The listing builds one solid part. Answer for the finished solid, in the listing's coordinates (mm). A direction names the side the tool comes from. Give positions to 0.01 mm unless a question says otherwise; leave off trailing zeros. Order: outer loops, then holes, each group sorted by start corner. A loop starts at its lowest first (then second) coordinate and runs counter-clockwise, first axis right, second up. Notation, with made-up numbers: (33.5, -37.75) - (44.5, -37.75) arc R30 cw to (44.5, -12.75) - close; hole circle Ø5 at (60, 80). An arc over 180 degrees is marked (long way). Use a Markdown table: item, result. Add a question column.
1) Find section B-B, the plane x = 13.5. Determine the outline of the cut face in (y, z) (3 decimals), plus the area to 3 significant figures.
2) Straight lines are drawn through the part: line 1 (X direction, y = 1.8, z = -4.65) (3 decimals); line 2 (Z direction, x = -4, y = 1.55) (3 decimals); line 3 (Z direction, x = 13.5, y = 1.65) (3 decimals). For each, find the intervals that lie inside material, in ascending order.
3) Find section C-C, the plane z = 30. Determine the outline of the cut face in (x, y).
4) The mould has two halves that part along X. Classify faces 4 (the face through (-2, 2, 31.5)), 5 (the face through (-14.448, 1.726, -22.078)), 6 (the face through (-14.853, 1.726, -3.946)): released by +X, released by -X, zero draft, split by the parting line, or undercut.
5) Find section A-A, the plane x = -13.5. Determine the outline of the cut face in (y, z) (3 decimals).
6) For faces 1 (the face through (-8.409, 1.774, -6.435)), 2 (the face through (-3.6, 2, 17)), 3 (the face through (19, 2, 15.4)), determine the directions among +Z, -Z, +X, -X, +Y, -Y from which every point of the face is accessible in a straight line to the end or side of a thin tool.
7) Find section D-D, the plane y = 0.8. State how many separate pieces and enclosed holes the cut face has, plus the area to 3 significant figures.
8) Flat-ended cylindrical pins translate along their axes: pin 1 (1 mm diameter, centred on y = 1.5, z = 14, fed in from -X); pin 2 (1.5 mm diameter, centred on y = 1.5, z = -16, fed in from +X); pin 3 (1.8 mm diameter, centred on x = 18.5, y = 1, fed in from -Z). Find the tip coordinate at first contact, or state that the pin passes through.
from build123d import *

# Parameters (mm, degrees)
SKETCH2_R           = 1.525
BOSS_EXTRUDE1_DEPTH = 3.5
FILLET1_R           = 5
FILLET2_R           = 2


with BuildPart() as part:
    # Sketch2 → Boss-Extrude1 (new body)
    with BuildSketch(Plane(origin=(0, 0, 0), x_dir=(1, 0, 0), z_dir=(0, 1, 0))):
        Polygon((-8, 29.459088021), (8, 29.459088021), (20.5, 15.15), (20.5, -13.4), (17, -13.4), (17, -15.4), (20.5, -15.4), (20.5, -18.9), (17, -18.9), (17, -31.5), (20.5, -31.5), (20.5, -35), (17, -35), (17, -37), (-0.1, -37), (-0.1, -35), (-3.6, -35), (-3.6, -31.5), (-0.1, -31.5), (-0.1, -18.9), (-3.6, -18.9), (-3.6, -15.4), (-0.1, -15.4), (-0.1, -13.4), (-3.6, -13.4), (-3.6, 0), (-20.5, 0), (-20.5, 15.15), align=None)
        with Locations(Location((-5.25, 25.459088021, 0), (0, 0, 270))):
            Circle(SKETCH2_R, mode=Mode.SUBTRACT)
        with Locations(Location((-13.5, 4.65, 0), (0, 0, 270))):
            Circle(SKETCH2_R, mode=Mode.SUBTRACT)
        with Locations(Location((13.5, 4.65, 0), (0, 0, 90))):
            Circle(SKETCH2_R, mode=Mode.SUBTRACT)
        with Locations(Location((5.25, 25.459088021, 0), (0, 0, 90))):
            Circle(SKETCH2_R, mode=Mode.SUBTRACT)
        with BuildLine():
            Line((8.711994152, 6.175), (-8.711994152, 6.175))
            ThreePointArc((-8.711994152, 6.175), (-10.168396205, 8.411786963), (-12.564791667, 9.587206738))
            ThreePointArc((-12.564791667, 9.587206738), (0, 18.15), (12.564791667, 9.587206738))
            ThreePointArc((12.564791667, 9.587206738), (10.168396205, 8.411786963), (8.711994152, 6.175))
        make_face(mode=Mode.SUBTRACT)
        with BuildLine():
            ThreePointArc((4.678763834, -20.194315192), (8.45, -25.527648525), (12.221236166, -20.194315192))
            ThreePointArc((12.221236166, -20.194315192), (8.45, -9.527648525), (4.678763834, -20.194315192))
        make_face(mode=Mode.SUBTRACT)
    extrude(amount=BOSS_EXTRUDE1_DEPTH)

    # Fillet1
    fillet1_edges = [part.edges().sort_by_distance(p)[0] for p in [
        (20.5, 1.75, -15.15),
        (-3.6, 1.75, 0),
        (-20.5, 1.75, 0),
        (-20.5, 1.75, -15.15),
        (-8, 1.75, -29.459088021),
        (8, 1.75, -29.459088021),
    ]]
    fillet(fillet1_edges, radius=FILLET1_R)

    # Fillet2
    fillet2_edges = [part.edges().sort_by_distance(p)[0] for p in [
        (-12.564791667, 1.75, -9.587206738),
        (-8.711994152, 1.75, -6.175),
        (8.711994152, 1.75, -6.175),
        (12.564791667, 1.75, -9.587206738),
    ]]
    fillet(fillet2_edges, radius=FILLET2_R)


solid = part.part
The answers:
| question | item | result |
|---|---|---|
| 1 | outline | (0, -23.163) - (3.5, -23.163) - (3.5, -6.175) - (0, -6.175) - close; (0, -3.125) - (3.5, -3.125) - (3.5, 12.288) - (0, 12.288) - close; (0, 18.768) - (3.5, 18.768) - (3.5, 37) - (0, 37) - close |
| 1 | area | 177 mm2 |
| 2 | line 1 | -20.488 to -15.025, -11.975 to 11.975, 15.025 to 20.5 |
| 2 | line 2 | -29.459 to -26.333, -24.586 to -17.544, -6.175 to 3.04 |
| 2 | line 3 | -23.163 to -6.175, -3.125 to 12.288, 18.768 to 37 |
| 3 | outline | (-0.1, 0) - (17, 0) - (17, 3.5) - (-0.1, 3.5) - close |
| 4 | face 4 | zero draft |
| 4 | face 5 | released by -X |
| 4 | face 6 | undercut |
| 5 | outline | (0, -23.163) - (3.5, -23.163) - (3.5, -6.175) - (0, -6.175) - close; (0, -3.125) - (3.5, -3.125) - (3.5, 0) - (0, 0) - close |
| 6 | face 1 | +Y, -Y |
| 6 | face 2 | +Z, -X, +Y, -Y |
| 6 | face 3 | +X, +Y, -Y |
| 7 | separate pieces | 1 |
| 7 | enclosed holes | 6 |
| 7 | area | 1,410 mm2 |
| 8 | pin 1 | x = -0.1 |
| 8 | pin 2 | x = 20.09 |
| 8 | pin 3 | z = -18.47 |
